Geometry: see drawing. Coordinates: mm, zero at the bounding-box minimum. A direction names the side the tool comes from. Give positions to 0.01 mm unless a question says otherwise; leave off trailing zeros. Write each loop counter-clockwise with the first axis right and the second up, starting at its lowest first coordinate (ties: lowest second). Pieces come first, ordered by that corner, then holes.
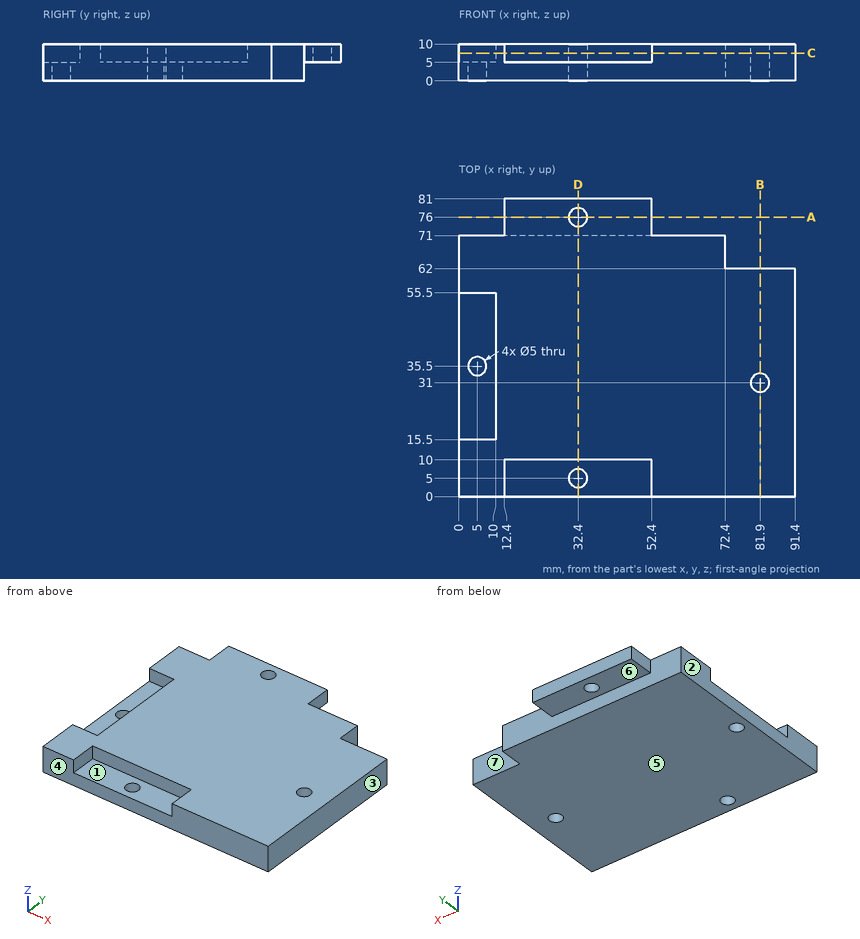
1. Line query: probe 1 along Y at (x, z) = (81.9, 4.75); probe 2 along Y at (x, z) = (32.4, 1.15); probe 3 along Z at (x, y) = (18.5, 75.5). Output: solid intervals per line, ascending.
2. Pin query (flat end, axial travel): P1, Ø2.5, axis at x = 5.5, z = 7.5, coming from the +Y side; P2, Ø8, axis at x = 32.4, y = 76, coming from the -Z side; P3, Ø8, axis at x = 34.5, y = 3, coming from the +Z side. Return the tip coordinate at first contact, or that it passes through.
3. Access query for the marked faces 5, 6 and 7. Directions: +Z, -Z, +X, -X, +Y, -Y. A direction counts if a zero-diameter tool reaches every point of the face in a straight line with its end or side. Return the directions, or none.
4. Section query A-A (y = 76). Return loops of the section in (x, z), plus the area to 3 significant figures.
5. Section query D-D (x = 32.4). Return loops of the section in (y, z).
6. Pull-direction query (X, two-part tool) for the marked faces 1, 2, 3 and 4; classes: pulls with the +X half, pulls with the -X half, needs draft (parallel to the pull), parting line crosses it, or undercut.
7. Section query C-C (z = 7.5). Return loops of the section in (x, y), plus the area to 3 significant figures.
8. Section query B-B (x = 81.9). Return loops of the section in (y, z).
The answers:
1. probe 1: y = 0 to 28.5, 33.5 to 62
1. probe 2: y = 0 to 2.5, 7.5 to 71
1. probe 3: z = 5 to 10
2. P1: stops at y = 71
2. P2: stops at z = 5
2. P3: stops at z = 5
3. face 5: -Z, +X, -X, +Y, -Y
3. face 6: -Z, +X, -X, +Y
3. face 7: +Z, -Z, +X, +Y
4. outline: (12.4, 5) - (29.9, 5) - (29.9, 10) - (12.4, 10) - close; (34.9, 5) - (52.4, 5) - (52.4, 10) - (34.9, 10) - close
4. area: 175 mm2
5. outline: (0, 0) - (2.5, 0) - (2.5, 5) - (0, 5) - close; (7.5, 0) - (71, 0) - (71, 5) - (73.5, 5) - (73.5, 10) - (10, 10) - (10, 5) - (7.5, 5) - close; (78.5, 5) - (81, 5) - (81, 10) - (78.5, 10) - close
6. face 1: undercut
6. face 2: pulls with the -X half
6. face 3: pulls with the +X half
6. face 4: needs draft
7. outline: (0, 0) - (12.4, 0) - (12.4, 10) - (52.4, 10) - (52.4, 0) - (91.4, 0) - (91.4, 62) - (72.4, 62) - (72.4, 71) - (52.4, 71) - (52.4, 81) - (12.4, 81) - (12.4, 71) - (0, 71) - (0, 55.5) - (10, 55.5) - (10, 15.5) - (0, 15.5) - close; hole circle Ø5 at (32.4, 76); hole circle Ø5 at (81.9, 31)
7. area: 5,880 mm2
8. outline: (0, 0) - (28.5, 0) - (28.5, 10) - (0, 10) - close; (33.5, 0) - (62, 0) - (62, 10) - (33.5, 10) - close
